The drawing under review shows one solid part. Ordinate dimensions are in mm from its lowest x, y, z. Round coordinates to 2 decimals unless told otherwise and drop trailing zeros. Order: outer loops, then holes, each group sorted by start corner. A loop starts at its lowest first (then second) coordinate and runs counter-clockwise, first axis right, second up. Notation, with made-up numbers: (-28, 33.5) -> (17, 33.5) arc R30 cw to (17, 58.5) -> close; hole circle Ø6 at (-35.75, -16). An arc over 180 degrees is marked (long way). Return JSON: item names as keys, results as strings. Group by question number.
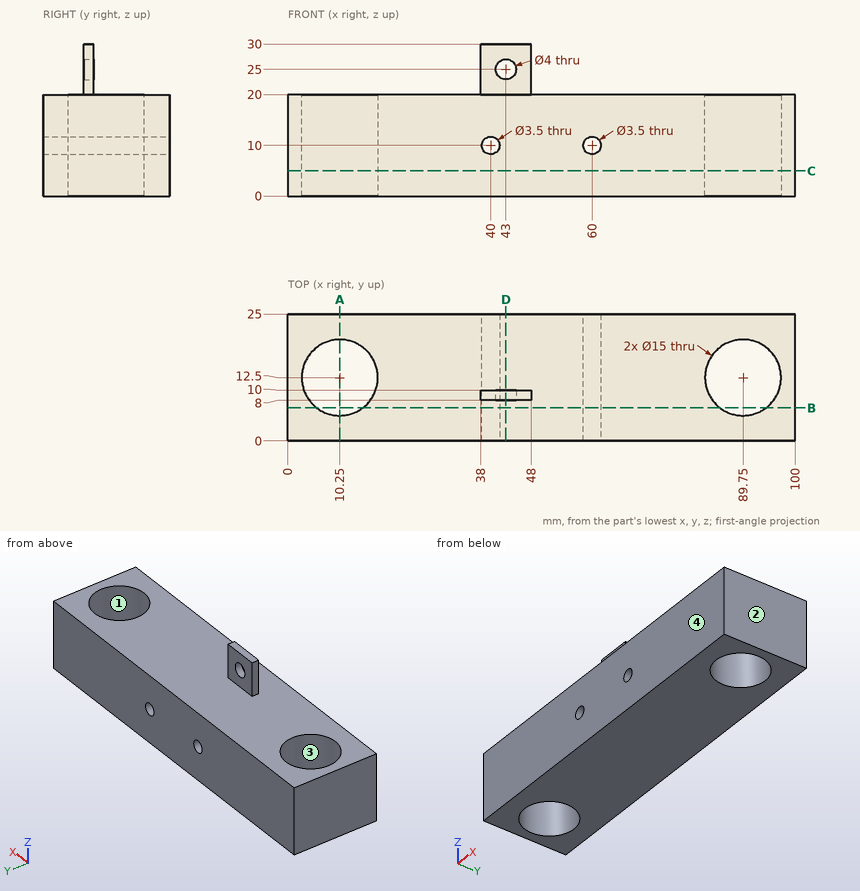
Item 1: Consider section C-C on z = 5. State the section outline as (x, y) points.
Item 2: Consider section A-A on x = 10.25. State the section outline as (y, z) points.
Item 3: Insertion check: pin 1 Ø5 at (x, z) = (45, 25.5) entering from +Y; pin 2 Ø1.6 at (y, z) = (8.5, 26) entering from -X; pin 3 Ø6 at (x, y) = (61.5, 9.5) entering from +Z; pin 4 Ø3 at (x, z) = (43, 25) entering from +Y. Each pin has a flat end and moves straight along its axis. Give the tip position at first contact, or say it passes through.
Item 4: Consider section B-B on y = 6.5. State the section outline as (x, z) points, plus the area to 3 significant figures.
Item 5: Consider section D-D on x = 43. State the section outline as (y, z) points.
Item 6: The part is to be moulded in two halves that separate along X. For the marked faces 1, 2, 3 and 4, say which applies: +X half, -X half, draft (parallel to the pull), parting line (faces both ways), or undercut.
Item 7: Wall thickness on line 1 along X through (y, z) = (17, 10); line 2 along X through (y, z) = (7.75, 8.5); line 3 along X through (y, z) = (6, 5): over which ranges is each line inside the solid? List them lowest first.
Values:
{
 "1": {"outline": "(0, 0) -> (100, 0) -> (100, 25) -> (0, 25) -> close; hole circle Ø15 at (10.25, 12.5); hole circle Ø15 at (89.75, 12.5)"},
 "2": {"outline": "(0, 0) -> (5, 0) -> (5, 20) -> (0, 20) -> close; (20, 0) -> (25, 0) -> (25, 20) -> (20, 20) -> close"},
 "3": {"pin 1": "y = 10", "pin 2": "x = 38", "pin 3": "z = 20", "pin 4": "through"},
 "4": {"outline": "(0, 0) -> (5.75, 0) -> (5.75, 20) -> (0, 20) -> close; (14.75, 0) -> (85.25, 0) -> (85.25, 20) -> (14.75, 20) -> close; (94.25, 0) -> (100, 0) -> (100, 20) -> (94.25, 20) -> close; hole circle Ø3.5 at (40, 10); hole circle Ø3.5 at (60, 10)", "area": "1,620 mm^2"},
 "5": {"outline": "(0, 0) -> (25, 0) -> (25, 20) -> (10, 20) -> (10, 23) -> (8, 23) -> (8, 20) -> (0, 20) -> close; (8, 27) -> (10, 27) -> (10, 30) -> (8, 30) -> close"},
 "6": {"face 1": "undercut", "face 2": "+X half", "face 3": "undercut", "face 4": "draft"},
 "7": {"line 1": "0 to 4.25, 16.25 to 38.25, 41.75 to 58.25, 61.75 to 83.75, 95.75 to 100", "line 2": "0 to 4.45, 16.05 to 39.1, 40.9 to 59.1, 60.9 to 83.95, 95.55 to 100", "line 3": "0 to 6.51, 13.99 to 86.01, 93.49 to 100"}
}
